Source: CAD feature listing. Evaluate the final solid. Frame: model axes, mm. A direction names the side the tool comes from. Coordinates: 2 decimals unless noted, no trailing zeros. Order: outer loops, then holes, each group sorted by start corner. A loop starts at its lowest first (then second) coordinate and runs counter-clockwise, first axis right, second up.
```python
from build123d import *

# Parameters (mm, degrees)
EXTRUDE_1_DEPTH      = 25
EXTRUDE_1_DEPTH_BACK = 25
SKETCH_2_W           = 5
SKETCH_2_H           = 12
EXTRUDE_2_DEPTH      = 20
SKETCH_3_R           = 4
CUT_EXTRUDE_1_DEPTH  = 41


with BuildPart() as part:
    # 草图1 → 凸台-拉伸1 (new, two sides: drawn at the far end of the back side and taken through both)
    with BuildSketch(Plane.XY.offset(-EXTRUDE_1_DEPTH_BACK)):
        Polygon((-12.553319429, 0), (5.446680571, 0), (5.446680571, 4), (-12.553319429, 4), (-12.553319429, 8), (8.446680571, 8), (8.446680571, -4), (-12.553319429, -4), align=None)
    extrude(amount=EXTRUDE_1_DEPTH + EXTRUDE_1_DEPTH_BACK)

    # 草图2 → 凸台-拉伸2 (add)
    with BuildSketch(Plane(origin=(8.446680571, 0, 0), x_dir=(0, 0, -1), z_dir=(1, 0, 0))):
        with Locations((-14.5, 2)):
            Rectangle(SKETCH_2_W, SKETCH_2_H)
        with Locations((14.5, 2)):
            Rectangle(SKETCH_2_W, SKETCH_2_H)
    extrude(amount=EXTRUDE_2_DEPTH)

    # 草图3 → 切除-拉伸1 (cut)
    with BuildSketch(Plane.XY.offset(17)):
        with Locations((21.446680571, 2)):
            Circle(SKETCH_3_R)
    extrude(amount=-CUT_EXTRUDE_1_DEPTH, mode=Mode.SUBTRACT)


solid = part.part
```
1. Section query C-C on z = -21. Return loops of the section in (x, y).
Findings:
outline: (-12.55, -4) - (8.45, -4) - (8.45, 8) - (-12.55, 8) - (-12.55, 4) - (5.45, 4) - (5.45, 0) - (-12.55, 0) - close
2. Section query D-D on x = 18.5. Return loops of the section in (y, z) (3 decimals), plus the area to 3 significant figures.
Findings:
outline: (-4, -17) - (-0.705, -17) - (-0.705, -12) - (-4, -12) - close; (-4, 12) - (-0.705, 12) - (-0.705, 17) - (-4, 17) - close; (4.705, -17) - (8, -17) - (8, -12) - (4.705, -12) - close; (4.705, 12) - (8, 12) - (8, 17) - (4.705, 17) - close
area: 65.9 mm2
3. Section query A-A on x = 2. Return loops of the section in (y, z).
Findings:
outline: (-4, -25) - (0, -25) - (0, 25) - (-4, 25) - close; (4, -25) - (8, -25) - (8, 25) - (4, 25) - close
4. Access query for faces 4 (the face through (8.447, 2, 0)), 5 (the face through (-4, 0, 0)), 6 (the face through (8.447, 2, -21)). Directions: +Z, -Z, +X, -X, +Y, -Y. A direction counts if a zero-diameter tool reaches every point of the face in a straight line with its end or side. Return the directions, or none.
Findings:
face 4: +X, +Y, -Y
face 5: +Z, -Z, -X
face 6: -Z, +X, +Y, -Y
5. Section query B-B on y = 2. Return loops of the section in (x, z), plus the area to 3 significant figures.
Findings:
outline: (5.45, -25) - (8.45, -25) - (8.45, -17) - (17.45, -17) - (17.45, -12) - (8.45, -12) - (8.45, 12) - (17.45, 12) - (17.45, 17) - (8.45, 17) - (8.45, 25) - (5.45, 25) - close; (25.45, -17) - (28.45, -17) - (28.45, -12) - (25.45, -12) - close; (25.45, 12) - (28.45, 12) - (28.45, 17) - (25.45, 17) - close
area: 270 mm2
6. Draft query along Y for faces 1 (the face through (25.262, 3.201, 14.535)), 2 (the face through (-1, 8, 0)), 3 (the face through (16, 2, 17)). Return one class per face: released by +Y, released by -Y, zero draft, split by the parting line, or undercut.
Findings:
face 1: undercut
face 2: released by +Y
face 3: zero draft
7. Ray query, line 1 (Y direction, x = 4.5, z = 21.5); line 2 (Z direction, x = 16.5, y = -0.25); line 3 (X direction, y = 1.5, z = 18). Return the intervals inside material, ascending.
Findings:
line 1: y = -4 to 0, 4 to 8
line 2: z = -17 to -12, 12 to 17
line 3: x = 5.45 to 8.45
8. Pin query (flat end, axial travel): P1, Ø3, axis at x = 18, y = 5.5, coming from the +Z side; P2, Ø2, axis at y = 1.5, z = -10, coming from the -X side; P3, Ø3.5, axis at x = 23, y = 0, coming from the -Z side. Return the tip coordinate at first contact, or that it passes through.
Findings:
P1: stops at z = 17
P2: stops at x = 5.45
P3: stops at z = -17
